from build123d import *

# Parameters (mm, degrees)
BOSS_EXTRUDE1_DEPTH = 1.2
BOSS_EXTRUDE2_DEPTH = 4.2
SKETCH3_W           = 5.20563433
SKETCH3_H           = 12.0272654
BOSS_EXTRUDE3_DEPTH = 14
CHAMFER3_SIZE       = 1
SKETCH4_W           = 5.20563433
SKETCH4_H           = 8.716640791
BOSS_EXTRUDE4_DEPTH = 5.4
BOSS_EXTRUDE5_DEPTH = 5.4
BOSS_EXTRUDE8_DEPTH = 5.4
FILLET1_R           = 2
FILLET3_R           = 1.4835
SKETCH12_R          = 31.501357271
CUT_EXTRUDE1_DEPTH  = 1


with BuildPart() as part:
    # Sketch1 → Boss-Extrude1 (new body)
    with BuildSketch(Plane(origin=(0, 0, 0), x_dir=(1, 0, 0), z_dir=(0, 1, 0))):
        Polygon((12.5, -19.496991909), (22.977471756, -2.044517527), (21.677471756, -2.044517527), (25.692225392, 4.642914958), (26.992225392, 4.642914958), (30, 9.653008091), (23.5, 20.103008091), (-23.5, 20.103008091), (-30, 9.653008091), (-26.992225392, 4.642914958), (-25.692225392, 4.642914958), (-21.677471756, -2.044517527), (-22.977471756, -2.044517527), (-12.5, -19.496991909), align=None)
        Polygon((-21.05511414, 15.703008091), (21.05511414, 15.703008091), (24.843569396, 9.612337718), (10.009495006, -15.096991909), (-10.009495006, -15.096991909), (-24.843569396, 9.612337718), align=None, mode=Mode.SUBTRACT)
    extrude(amount=BOSS_EXTRUDE1_DEPTH)

    # Sketch2 → Boss-Extrude2 (add)
    with BuildSketch(Plane(origin=(0, 1.2, 0), x_dir=(1, 0, 0), z_dir=(0, 1, 0))):
        Polygon((26.71863507, 9.627126944), (21.944163543, 17.303008091), (-21.944163543, 17.303008091), (-26.71863507, 9.627126944), (-10.915133186, -16.696991909), (10.915133186, -16.696991909), align=None)
        Polygon((24.843569396, 9.612337718), (21.05511414, 15.703008091), (-21.05511414, 15.703008091), (-24.843569396, 9.612337718), (-10.009495006, -15.096991909), (10.009495006, -15.096991909), align=None, mode=Mode.SUBTRACT)
    extrude(amount=BOSS_EXTRUDE2_DEPTH)

    # Sketch3 → Boss-Extrude3 (add)
    with BuildSketch(Plane.XZ):
        with Locations((0, -13)):
            Rectangle(SKETCH3_W, SKETCH3_H)
    extrude(amount=BOSS_EXTRUDE3_DEPTH)

    # Chamfer3
    chamfer3_edges = [part.edges().sort_by_distance(p)[0] for p in [
        (0, 0, -19.0136327),
    ]]
    chamfer(chamfer3_edges, length=CHAMFER3_SIZE)

    # Sketch4 → Boss-Extrude4 (add)
    with BuildSketch(Plane(origin=(0, 0, 0), x_dir=(1, 0, 0), z_dir=(0, 1, 0))):
        with Locations((0, 11.344687696)):
            Rectangle(SKETCH4_W, SKETCH4_H)
    extrude(amount=BOSS_EXTRUDE4_DEPTH)

    # Sketch6 → Boss-Extrude5 (add)
    with BuildSketch(Plane(origin=(0, 5.4, 0), x_dir=(1, 0, 0), z_dir=(0, 1, 0))):
        Polygon((-7.835791911, 15.703008091), (-2.602817165, 6.9863673), (-2.602817165, 15.703008091), align=None)
    boss_extrude5 = extrude(amount=-BOSS_EXTRUDE5_DEPTH)

    # Mirror1: Boss-Extrude5 across plane
    add(boss_extrude5.mirror(Plane(origin=(0, 0, 0), x_dir=(0, 0, 1), z_dir=(1, 0, 0))))

    # Sketch10 → Boss-Extrude8 (add)
    with BuildSketch(Plane(origin=(0, 0, 0), x_dir=(-1, 0, 0), z_dir=(0, -1, 0))):
        Polygon((-2.602817165, 6.9863673), (-4.146953179, 9.558456717), (-17.976484501, -1.826263693), (-16.432348487, -4.398353111), align=None)
        Polygon((2.602817165, 6.9863673), (4.146953179, 9.558456717), (17.976484501, -1.826263693), (16.432348487, -4.398353111), align=None)
    extrude(amount=-BOSS_EXTRUDE8_DEPTH)

    # Fillet1
    fillet1_edges = [part.edges().sort_by_distance(p)[0] for p in [
        (-7.835791911, 2.7, -15.703008091),
        (7.835791911, 2.7, -15.703008091),
        (4.146953179, 2.7, -9.558456717),
        (17.976484501, 2.7, 1.826263693),
        (16.432348487, 2.7, 4.398353111),
        (-17.976484501, 2.7, 1.826263693),
        (-4.146953179, 2.7, -9.558456717),
        (-16.432348487, 2.7, 4.398353111),
        (10.009495006, 2.7, 15.096991909),
        (24.843569396, 2.7, -9.612337718),
        (21.05511414, 2.7, -15.703008091),
        (-21.05511414, 2.7, -15.703008091),
        (-24.843569396, 2.7, -9.612337718),
        (-10.009495006, 2.7, 15.096991909),
    ]]
    fillet(fillet1_edges, radius=FILLET1_R)

    # Fillet3
    fillet3_edges = [part.edges().sort_by_distance(p)[0] for p in [
        (-8.852151276, 0, -1.841802387),
        (-13.068628591, 0, 10.001349395),
        (13.068628591, 0, 10.001349395),
        (8.852151276, 0, -1.841802387),
        (0, 0, 15.096991909),
        (-14.45582101, 0, -15.703008091),
        (-22.920045025, 0, -12.704773052),
        (-21.692654112, 0, -4.363813116),
        (-10.831403301, 0, -4.055696431),
        (-6.143665701, 0, -12.88440929),
        (6.143665701, 0, -12.88440929),
        (14.45582101, 0, -15.703008091),
        (22.920045025, 0, -12.704773052),
        (21.692654112, 0, -4.363813116),
        (10.831403301, 0, -4.055696431),
        (-15.801291957, 0, 4.507128455),
        (15.801291957, 0, 4.507128455),
        (9.862625433, 0, 14.837515971),
        (-9.862625433, 0, 14.837515971),
        (-20.915222266, 0, -15.451248181),
        (-24.499675096, 0, -9.609625316),
        (-17.795848772, 0, 0.778311547),
        (-7.982661484, 0, -15.443532153),
        (7.982661484, 0, -15.443532153),
        (20.915222266, 0, -15.451248181),
        (24.499675096, 0, -9.609625316),
        (17.795848772, 0, 0.778311547),
        (4.778009709, 0, -9.667232062),
        (-4.778009709, 0, -9.667232062),
    ]]
    fillet(fillet3_edges, radius=FILLET3_R)

    # Sketch12 → Cut-Extrude1 (cut)
    with BuildSketch(Plane(origin=(0, 5.4, 0), x_dir=(1, 0, 0), z_dir=(0, 1, 0))):
        Circle(SKETCH12_R)
    extrude(amount=-CUT_EXTRUDE1_DEPTH, mode=Mode.SUBTRACT)


solid = part.part
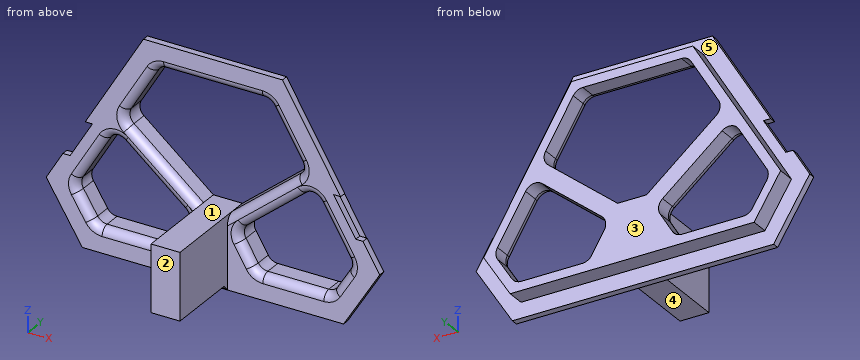
Source: CAD feature listing. Evaluate the final solid. Frame: model axes, mm. Face numbers are marked on the shaded views. A direction names the side the tool comes from. Coordinates: 2 decimals unless noted, no trailing zeros. Write each loop counter-clockwise with the first axis right and the second up, starting at its lowest first coordinate (ties: lowest second). Pieces come first, ordered by that corner, then holes. Notation, with made-up numbers: M -39,63 L 13,63 A18 ccw 13,72 Z; hole C 22,-16.75 d10. An arc over 180 degrees is marked long. Use a Markdown table: item, result.
1) Ray query, L1, parallel to X at y = 1.5, z = -10; L2, parallel to X at y = 3, z = -11; L3, parallel to Y at x = -15.5, z = -16. Return the intervals inside material, ascending.
Conclusion:
| item | result |
|---|---|
| L1 | x = -26.49 to -24.46, -4.75 to 4.75, 24.46 to 26.49 |
| L2 | x = -25.86 to -23.98, -5.01 to 5.01, 23.98 to 25.86 |
| L3 | y = 0.59 to 4.4 |
2) Section B-B, the plane y = -2.25. Output: boundary loops of the cut face in (x, z), then the cut area to 3 significant figures.
Conclusion:
| item | result |
|---|---|
| outline | M -2.6,-19.01 L 2.6,-19.01 L 2.6,-6.99 L -2.6,-6.99 Z |
| area | 62.6 mm^2 |
3) Reachability of the marked faces 3, 4 and 5 from +Z, -Z, +X, -X, +Y, -Y: full face, straight path, thin tool, end or side. Return the list, or none.
Conclusion:
| item | result |
|---|---|
| face 3 | +Z, -Z, +X, -X, +Y |
| face 4 | -Z, +X, -X, -Y |
| face 5 | +Y |
4) First-contact query: pin 1 Ø1.3 at (x, y) = (-26.5, 0.5) entering from +Z; pin 2 Ø0.9 at (x, y) = (12.5, 2.5) entering from +Z; pin 3 Ø4 at (y, z) = (-9, -14) entering from -X. Flat tips, straight axial feed; report the tip coordinate or a pass-through.
Conclusion:
| item | result |
|---|---|
| pin 1 | stops at z = -4.64 |
| pin 2 | stops at z = 14.81 |
| pin 3 | stops at x = -2.6 |
5) Mould query, pull axis X, two halves, no side actions, for the marked faces 1 and 2. Classes: pulls with the +X half, pulls with the -X half, needs draft (parallel to the pull), parting line crosses it, or undercut.
Conclusion:
| item | result |
|---|---|
| face 1 | undercut |
| face 2 | needs draft |
6) Section A-A, the plane z = -1.5. Give the number of separate pieces and of enclosed holes in the cut face, then the cut area to 3 significant figures.
Conclusion:
| item | result |
|---|---|
| separate pieces | 4 |
| enclosed holes | 0 |
| area | 58.1 mm^2 |
